from build123d import *

# Parameters (mm, degrees)
BOSS_EXTRUDE1_DEPTH           = 24
SKETCH6_W                     = 30
SKETCH6_H                     = 4
CUT_EXTRUDE2_DEPTH            = 286.642446166
CUT_EXTRUDE1_DEPTH            = 242.081568844
SKETCH7_R                     = 1.5
BOSS_EXTRUDE2_DEPTH           = 8
BOSS_EXTRUDE2_DRAFT           = 10
BOSS_EXTRUDE2_PROFILE_2_DEPTH = 8
BOSS_EXTRUDE2_PROFILE_2_DRAFT = 10


with BuildPart() as part:
    # Sketch4 → Boss-Extrude1 (new, symmetric)
    with BuildSketch(Plane(origin=(-229.78233317, -228.51233317, 0), x_dir=(0, 1, 0), z_dir=(0, 0, 1))):
        Polygon((-0.84773851, -8.551941602), (0.807370009, -7.949531351), (0.807370009, -7.269034775), (-0.84773851, -6.666624604), (-0.84773851, -6.01679977), (0.807370009, -5.414389518), (0.807370009, -4.733892942), (-0.84773851, -4.131482772), (-0.84773851, -3.481657937), (0.807370009, -2.879247686), (0.807370009, -2.19875111), (-0.84773851, -1.596340939), (-0.84773851, -0.946516105), (0.807370009, -0.344105854), (0.807370009, 0.336390722), (-0.84773851, 0.938800893), (-0.84773851, 1.588625727), (0.807370009, 2.191035978), (0.807370009, 2.871532554), (-0.84773851, 3.473942725), (-0.84773851, 4.123767559), (0.807370009, 4.726177811), (0.807370009, 5.406674387), (-0.84773851, 6.009084557), (-0.84773851, 6.658909392), (0.807370009, 7.261319643), (0.807370009, 7.941816219), (-0.84773851, 8.54422639), (-0.84773851, 9.194051224), (0.807370009, 9.796461475), (0.807370009, 10.476958051), (-0.84773851, 11.079368222), (-0.84773851, 11.729193056), (0.807370009, 12.331603308), (0.807370009, 13.012099883), (-0.84773851, 13.614510054), (-0.84773851, 14.264334888), (0.807370009, 14.86674514), (0.807370009, 15.547241716), (-0.84773851, 16.149651886), (-0.84773851, 16.799476721), (0.807370009, 17.401886972), (0.807370009, 18.082383548), (-0.84773851, 18.684793719), (-0.84773851, 19.334618553), (0.807370009, 19.937028804), (0.807370009, 20.61752538), (-0.84773851, 21.219935551), (-0.84773851, 21.869760385), (0.807370009, 22.472170637), (0.807370009, 23.152667212), (-0.84773851, 23.755077383), (-0.84773851, 24.404902217), (0.807370009, 25.007312469), (0.807370009, 25.687809045), (-0.84773851, 26.290219215), (-0.84773851, 26.94004405), (0.807370009, 27.542454301), (0.807370009, 28.222950877), (-0.84773851, 28.825361048), (-0.84773851, 29.475185882), (0.807370009, 30.077596133), (0.807370009, 30.758092709), (-0.84773851, 31.36050288), (-0.84773851, 32.010327714), (0.807370009, 32.612737966), (0.807370009, 33.293234541), (-0.84773851, 33.895644712), (-0.84773851, 34.545469546), (0.807370009, 35.147879798), (0.807370009, 35.828376374), (-0.84773851, 36.430786544), (-0.84773851, 37.080611379), (0.807370009, 37.68302163), (0.807370009, 38.363518206), (-0.84773851, 38.965928377), (-0.84773851, 39.615753211), (0.807370009, 40.218163462), (0.807370009, 40.898660038), (-0.84773851, 41.501070209), (-0.84773851, 42.150895043), (0.807370009, 42.753305295), (0.807370009, 43.43380187), (-0.84773851, 44.036212041), (-0.84773851, 44.686036875), (0.807370009, 45.288447127), (0.807370009, 45.968943703), (-0.84773851, 46.571353873), (-0.84773851, 47.221178708), (0.807370009, 47.823588959), (0.807370009, 48.504085535), (-0.84773851, 49.106495706), (-0.84773851, 49.75632054), (0.807370009, 50.358730791), (0.807370009, 51.039227367), (-0.84773851, 51.641637538), (-0.84773851, 52.291462372), (0.807370009, 52.893872624), (0.807370009, 53.574369199), (-0.84773851, 54.17677937), (-0.84773851, 54.826604204), (-2.84773851, 54.826604204), (-2.84773851, -8.551941602), align=None)
    extrude(amount=BOSS_EXTRUDE1_DEPTH, both=True)

    # Sketch6 → Cut-Extrude2 (cut, through all)
    with BuildSketch(Plane.XZ.offset(231.36007168)):
        with Locations((-269.608937374, -22)):
            Rectangle(SKETCH6_W, SKETCH6_H)
        with Locations((-269.608937374, 22)):
            Rectangle(SKETCH6_W, SKETCH6_H)
    extrude(amount=-CUT_EXTRUDE2_DEPTH, mode=Mode.SUBTRACT)

    # Sketch5 → Cut-Extrude1 (cut, through all)
    with BuildSketch(Plane(origin=(-221.230391568, 0, 0), x_dir=(0, 0, -1), z_dir=(1, 0, 0))):
        with BuildLine():
            Line((-22.17244574, -227.704963161), (-22.17244574, -227.204963161))
            Line((-22.17244574, -227.204963161), (-24.67244574, -227.204963161))
            Line((-24.67244574, -227.204963161), (-24.67244574, -231.86007168))
            Line((-24.67244574, -231.86007168), (-22.17244574, -231.86007168))
            Line((-22.17244574, -231.86007168), (-22.17244574, -231.36007168))
            ThreePointArc((-22.17244574, -231.36007168), (-24, -229.53251742), (-22.17244574, -227.704963161))
        make_face()
        with BuildLine():
            Line((22.17244574, -231.86007168), (22.17244574, -231.36007168))
            ThreePointArc((22.17244574, -231.36007168), (24, -229.53251742), (22.17244574, -227.704963161))
            Line((22.17244574, -227.704963161), (22.17244574, -227.204963161))
            Line((22.17244574, -227.204963161), (24.67244574, -227.204963161))
            Line((24.67244574, -227.204963161), (24.67244574, -231.86007168))
            Line((24.67244574, -231.86007168), (22.17244574, -231.86007168))
        make_face()
    extrude(amount=-CUT_EXTRUDE1_DEPTH, mode=Mode.SUBTRACT)


with BuildPart() as boss_extrude2_tool:
    # Sketch7 → Boss-Extrude2 (with draft: the straight prism first)
    with BuildSketch(Plane.XZ.offset(231.36007168)):
        with Locations((-229.230391568, -15.991845927)):
            Circle(SKETCH7_R)
    extrude(amount=-BOSS_EXTRUDE2_DEPTH)
    # Boss-Extrude2: the draft: its side faces are tilted about the plane it starts from
    boss_extrude2_sides = [boss_extrude2_tool.faces().sort_by_distance(p)[0] for p in [
        (-230.730391568, -227.36007168, -15.991845927),
    ]]
    draft(boss_extrude2_sides, Plane.XZ.offset(231.36007168), BOSS_EXTRUDE2_DRAFT)


with BuildPart() as part_1:
    add(part.part)

    # Boss-Extrude2: add boss_extrude2_tool
    add(boss_extrude2_tool.part)


with BuildPart() as boss_extrude2_profile_2_tool:
    # Sketch7 → Boss-Extrude2 profile 2 (with draft: the straight prism first)
    with BuildSketch(Plane.XZ.offset(231.36007168)):
        with Locations((-229.230391568, 15.991845927)):
            Circle(SKETCH7_R)
    extrude(amount=-BOSS_EXTRUDE2_PROFILE_2_DEPTH)
    # Boss-Extrude2 profile 2: the draft: its side faces are tilted about the plane it starts from
    boss_extrude2_profile_2_sides = [boss_extrude2_profile_2_tool.faces().sort_by_distance(p)[0] for p in [
        (-230.730391568, -227.36007168, 15.991845927),
    ]]
    draft(boss_extrude2_profile_2_sides, Plane.XZ.offset(231.36007168), BOSS_EXTRUDE2_PROFILE_2_DRAFT)


with BuildPart() as part_2:
    add(part_1.part)

    # Boss-Extrude2 profile 2: add boss_extrude2_profile_2_tool
    add(boss_extrude2_profile_2_tool.part)


solid = part_2.part
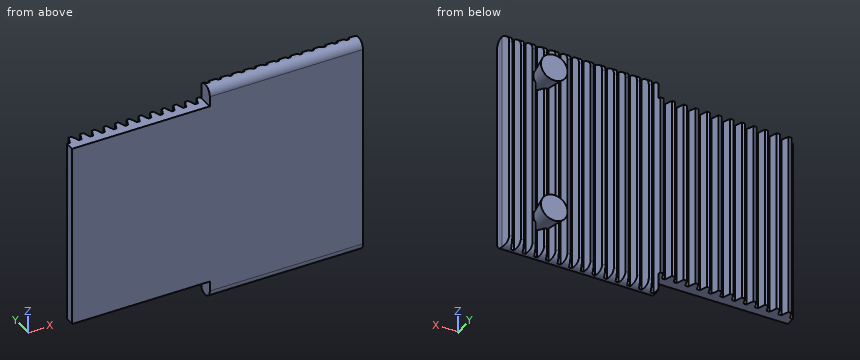
Check sheet for the modelled part. Datum: model origin and axes. Units: mm. Round coordinates to 2 decimals unless told otherwise and drop trailing zeros. Loops run counter-clockwise (first coordinate to the right, second up) from the corner with the lowest first, then second, coordinate; pieces in that order, holes last. Notation, with made-up numbers: M 71.25,-35.75 L 85.25,-35.75 A18 cw 85.25,-22.75 Z; hole C 11.25,-29.75 d11. An arc over 180 degrees is marked long. One line per item, written item: value.
(1) Sectioned sample at B-B, the plane y = -230.5. Record the cut outline in (x, z).
Computed values:
outline: M -284.61,-20 L -254.61,-20 L -254.61,-23.72 L -221.23,-23.72 L -221.23,23.72 L -254.61,23.72 L -254.61,20 L -284.61,20 Z
(2) Sectioned sample at A-A, the plane y = -225.75. Record the cut outline in (x, z).
Computed values:
outline: C -229.23,-15.99 d4.98; C -229.23,15.99 d4.98
(3) Thickness scan on line 1 (Y direction, x = -236, z = -0.5); line 2 (Z direction, x = -231, y = -225.5); line 3 (Z direction, x = -265.5, y = -229.25). Record the ranges inside material, lowest first.
Computed values:
line 1: y = -231.36 to -229.36
line 2: z = -17.8 to -14.18, 14.18 to 17.8
line 3: z = -20 to 20
(4) Depth check by flat-ended pin: pin 1 Ø0.7 at (x, z) = (-232.5, -5.5) entering from +Y; pin 2 Ø1 at (x, y) = (-272.5, -229) entering from -Z. Enter the tip coordinate at first touch or a pass-through.
Computed values:
pin 1: stops at y = -227.7
pin 2: stops at z = -20
